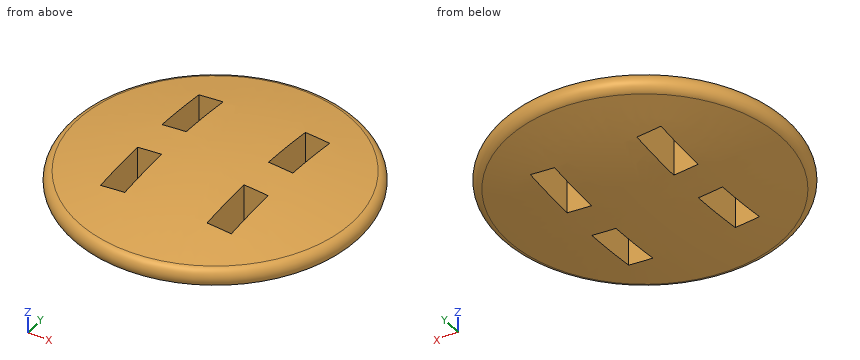
```python
from build123d import *

# Parameters (mm, degrees)
F2_W             = 50
F2_H             = 120
F3_DEPTH         = 50.001
F3_DEPTH_BACK    = 50.001
F3_COPIES2_COUNT = 2


# Not quite as in the source:
# - a pattern or mirror of a feature is missing from the dataset's text; its kind, count and spacing are read off the source's solid


with BuildPart() as f1:
    # F0 (on Front) → F1 (revolve)
    with BuildSketch(Plane.XZ):
        with BuildLine():
            ThreePointArc((284.237074401, -19.5460277427), (300, 0), (284.237074401, 19.5460277427))
            ThreePointArc((284.237074401, 19.5460277427), (142.931940876, 42.3647815091), (0, 50))
            Line((0, 50), (0, -50))
            ThreePointArc((0, -50), (142.931940876, -42.3647815091), (284.237074401, -19.5460277428))
        make_face()
    revolve(axis=Axis((0, 0, 0), (0, 0, -1)))

    # F2 (on Top) → F3 (cut, two sides)
    with BuildSketch(Plane.XY) as f3_sk:
        with Locations((-110, 100)):
            Rectangle(F2_W, F2_H)
    f3 = extrude(amount=-F3_DEPTH, mode=Mode.SUBTRACT) + extrude(f3_sk.sketch, amount=F3_DEPTH_BACK, mode=Mode.SUBTRACT)

    # F3_copies: F3 across plane
    add(f3.mirror(Plane(origin=(0, 0, 0), x_dir=(0, 0, 1), z_dir=(1, 0, 0))), mode=Mode.SUBTRACT)

    # F3_copies1: F3 across plane
    add(f3.mirror(Plane(origin=(0, 0, 0), x_dir=(0, 0, -1), z_dir=(0, -1, 0))), mode=Mode.SUBTRACT)

    # F3_copies2: F3 ×2 about axis
    f3_copies2_axis = Axis((0, 0, 0), (0, 0, 1))
    for i in range(1, F3_COPIES2_COUNT):
        add(f3.rotate(f3_copies2_axis, i * 360 / F3_COPIES2_COUNT), mode=Mode.SUBTRACT)


solid = f1.part
```
Input: part model. Units: mm. Frame: model coordinates. Give positions to 0.01 mm unless a question says otherwise; leave off trailing zeros. Order: outer loops, then holes, each group sorted by start corner. A loop starts at its lowest first (then second) coordinate and runs counter-clockwise, first axis right, second up. Notation, with made-up numbers: (-2.5, -27) - (31.5, -27) arc R22 cw to (31.5, 7) - close; hole circle Ø2 at (70, -17). An arc over 180 degrees is marked (long way). One line per item, written item: value.
1. Line query: probe 1 along Z at (x, y) = (52.5, -78); probe 2 along Z at (x, y) = (-135, 192.5); probe 3 along Y at (x, z) = (26, 3). Output: solid intervals per line, ascending.
Determined:
probe 1: -46.7 to 46.7
probe 2: -29.24 to 29.24
probe 3: -298.64 to 298.64
2. Cut plane A-A, the plane z = 0. Output: boundary loops of the cut face in (x, y).
Determined:
outline: circle Ø600 at (0, 0); hole (-135, -160) - (-85, -160) - (-85, -40) - (-135, -40) - close; hole (-135, 40) - (-85, 40) - (-85, 160) - (-135, 160) - close; hole (85, -160) - (135, -160) - (135, -40) - (85, -40) - close; hole (85, 40) - (135, 40) - (135, 160) - (85, 160) - close
3. Pin query (flat end, axial travel): pin 1 Ø5 at (y, z) = (-170.5, -18) entering from -X; pin 2 Ø15 at (x, z) = (121.5, -8.5) entering from +Y; pin 3 Ø2 at (x, y) = (87.5, 168) entering from +Z. Return the tip coordinate at first contact, or that it passes through.
Determined:
pin 1: x = -238.23
pin 2: y = 276.46
pin 3: z = 36.7
4. Cut plane B-B, the plane x = -112.5. Give the number of separate pieces and of enclosed holes in the cut face, and give its area (3 significant figures).
Determined:
separate pieces: 3
enclosed holes: 0
area: 19,600 mm2
